```python
from build123d import *

# Parameters (mm, degrees)
F0_W     = 4.2475935817
F0_H     = 4.5055083651
F0_W_2   = 5
F0_H_2   = 5
F1_DEPTH = 350
F2_ANGLE = 90


with BuildPart() as f1:
    # F0 (on Front) → F1 (new body)
    with BuildSketch(Plane.XZ):
        with BuildLine():
            Line((-43.9187724888, 48.8732061069), (-50.9187724888, 48.8732061069))
            ThreePointArc((-50.9187724888, 48.8732061069), (-53.0400928324, 47.9945264505), (-53.9187724888, 45.8732061069))
            Line((-53.9187724888, 45.8732061069), (-53.9187724888, 38.8732061069))
            Line((-53.9187724888, 38.8732061069), (-48.9187724888, 38.8732061069))
            Line((-48.9187724888, 38.8732061069), (-43.9187724888, 38.8732061069))
            Line((-43.9187724888, 38.8732061069), (-43.9187724888, 43.3787144721))
            Line((-43.9187724888, 43.3787144721), (-43.9187724888, 48.8732061069))
        make_face()
        with Locations((-41.794975698, 41.1259602895)):
            Rectangle(F0_W, F0_H)
        with Locations((-46.4187724888, 36.3732061069)):
            Rectangle(F0_W_2, F0_H_2)
    extrude(amount=F1_DEPTH)

    # F0 (on Front) → F2 (revolve)
    with BuildSketch(Plane.XZ):
        with BuildLine():
            Line((-43.9187724888, 48.8732061069), (-50.9187724888, 48.8732061069))
            ThreePointArc((-50.9187724888, 48.8732061069), (-53.0400928324, 47.9945264505), (-53.9187724888, 45.8732061069))
            Line((-53.9187724888, 45.8732061069), (-53.9187724888, 38.8732061069))
            Line((-53.9187724888, 38.8732061069), (-48.9187724888, 38.8732061069))
            Line((-48.9187724888, 38.8732061069), (-43.9187724888, 38.8732061069))
            Line((-43.9187724888, 38.8732061069), (-43.9187724888, 43.3787144721))
            Line((-43.9187724888, 43.3787144721), (-43.9187724888, 48.8732061069))
        make_face()
        with Locations((-41.794975698, 41.1259602895)):
            Rectangle(F0_W, F0_H)
        with Locations((-46.4187724888, 36.3732061069)):
            Rectangle(F0_W_2, F0_H_2)
    revolve(axis=Axis((-39.6711789072, 0, 41.1259602895), (0, 0, -1)), revolution_arc=F2_ANGLE)


solid = f1.part
```
Source: CAD feature listing. Evaluate the final solid. Frame: model axes, mm. A direction names the side the tool comes from. Round coordinates to 2 decimals unless told otherwise and drop trailing zeros. Loops run counter-clockwise (first coordinate to the right, second up) from the corner with the lowest first, then second, coordinate; pieces in that order, holes last. Notation, with made-up numbers: (30.25, 19.25) - (80.25, 19.25) arc R31 cw to (80.25, 47.25) - close; hole circle Ø11 at (22, 54.25). An arc over 180 degrees is marked (long way). Use CSV: the item, a comma, the result in double quotes.
Q1. Section query A-A, the plane y = -30.5. Output: boundary loops of the cut face in (x, z), then the cut area to 3 significant figures.
Reported:
outline,"(-53.92, 38.87) - (-48.92, 38.87) - (-48.92, 33.87) - (-43.92, 33.87) - (-43.92, 38.87) - (-39.67, 38.87) - (-39.67, 43.38) - (-43.92, 43.38) - (-43.92, 48.87) - (-50.92, 48.87) arc R3 ccw to (-53.92, 45.87) - close"
area,"142 mm^2"
Q2. Ray query, line 1 along X through (y, z) = (-209.5, 45); line 2 along Z through (x, y) = (-51.25, -2); line 3 along X through (y, z) = (-119.5, 35.5). Return the intervals inside material, ascending.
Reported:
line 1,"-53.92 to -43.92"
line 2,"38.87 to 48.85"
line 3,"-48.92 to -43.92"
Q3. Pin query (flat end, axial travel): pin 1 Ø1.3 at (x, y) = (-42.5, -238.5) entering from +Z; pin 2 Ø4.5 at (x, y) = (-41.5, -219) entering from -Z; pin 3 Ø2.5 at (y, z) = (-185.5, 35.5) entering from -X. Return the tip coordinate at first contact, or that it passes through.
Reported:
pin 1,"z = 43.38"
pin 2,"z = 38.87"
pin 3,"x = -48.92"
Q4. Section query B-B, the plane z = 36.25. Output: boundary loops of the cut face in (x, y).
Reported:
outline,"(-48.92, -350) - (-43.92, -350) - (-43.92, 0) arc R4.25 cw to (-39.67, 4.25) - (-39.67, 9.25) arc R9.25 ccw to (-48.92, 0) - close"
Q5. Reachability of faces 1 (the flat face through (-47, -350, 41)), 2 (the cylindrical face through (-46.28, 6.47, 36.41)), 3 (the flat face through (-43.919, -173, 46)) from +Z, -Z, +X, -X, +Y, -Y: full face, straight path, thin tool, end or side. Return the list, or none.
Reported:
face 1,"+Z, -Z, +X, -X, -Y"
face 2,"-Z, -X, +Y"
face 3,"+Z, +X, -Y"
